Read the model definition and answer for the solid it produces. Units are mm, in the model's axes. A direction names the side the tool comes from. Coordinates: 2 decimals unless noted, no trailing zeros. Order: outer loops, then holes, each group sorted by start corner. A loop starts at its lowest first (then second) coordinate and runs counter-clockwise, first axis right, second up. Notation, with made-up numbers: (61.25, 48.5) - (83.25, 48.5) arc R28 ccw to (83.25, 80.5) - close; hole circle Ø10 at (20, -11.75). An arc over 180 degrees is marked (long way). Use one line per item in the form item = value. Start each with the question number.
from build123d import *

# Parameters (mm, degrees)
F1_W     = 57.62729
F1_H     = 2.417922
F2_DEPTH = 53.739645
F3_W     = 20.9051
F3_H     = 3.238531
F4_DEPTH = 25
F5_W     = 39.400994
F5_H     = 8.231058
F6_DEPTH = 25


with BuildPart() as f2:
    # F1 (on face) → F2 (new body)
    with BuildSketch(Plane.XZ):
        with Locations((0, 114.370458)):
            Rectangle(F1_W, F1_H)
    extrude(amount=F2_DEPTH)

    # F3 (on face) → F4 (cut)
    with BuildSketch(Plane.XY.offset(115.579419)):
        with Locations((0, -6.892247)):
            Rectangle(F3_W, F3_H)
    extrude(amount=-F4_DEPTH, mode=Mode.SUBTRACT)

    # F5 (on face) → F6 (cut)
    with BuildSketch(Plane.XZ):
        with Locations((0, -5.288288)):
            Rectangle(F5_W, F5_H)
    extrude(amount=F6_DEPTH, mode=Mode.SUBTRACT)


solid = f2.part
Q1. A cutting plane is placed at C-C (z = 113.65). Give the vertices of the cut face in (x, y), then the cut area to 3 significant figures.
Q2. Consider probe 1 along Y at (x, z) = (-8, 113.75); probe 2 along X at (y, z) = (-7, 115). Determine where each line is inside the solid, lowest interval first.
Q3. Which of the six approach directions +Z, -Z, +X, -X, +Y, -Y give full straight-line access (tool end or side, diameter ignored) to faces 4 (the flat face through (0, -26, 113.161)), 5 (the flat face through (0, -5.273, 114))?
Q4. For a pull along X with two mould halves and no side action, classify faces 1 (the flat face through (-28.814, -26, 114)), 2 (the flat face through (0, -53.74, 114)), 3 (the flat face through (10.453, -7, 114)) as +X half, -X half, draft (parallel to the pull), parting line (faces both ways), or undercut.
Q5. A cutting plane is placed at A-A (x = 0). Give the vertices of the cut face in (y, z).
Q6. A cutting plane is placed at B-B (y = -6). Give the vertices of the cut face in (x, z), then the cut area to 3 significant figures.
Result sheet:
q1.outline = (-28.81, -53.74) - (28.81, -53.74) - (28.81, 0) - (-28.81, 0) - close; hole (-10.45, -8.51) - (10.45, -8.51) - (10.45, -5.27) - (-10.45, -5.27) - close
q1.area = 3,030 mm^2
q2.probe_1 = -53.74 to -8.51, -5.27 to 0
q2.probe_2 = -28.81 to -10.45, 10.45 to 28.81
q3.face_4 = -Z, +X, -X, +Y, -Y
q3.face_5 = +Z, -Z
q4.face_1 = -X half
q4.face_2 = draft
q4.face_3 = undercut
q5.outline = (-53.74, 113.16) - (-8.51, 113.16) - (-8.51, 115.58) - (-53.74, 115.58) - close; (-5.27, 113.16) - (0, 113.16) - (0, 115.58) - (-5.27, 115.58) - close
q6.outline = (-28.81, 113.16) - (-10.45, 113.16) - (-10.45, 115.58) - (-28.81, 115.58) - close; (10.45, 113.16) - (28.81, 113.16) - (28.81, 115.58) - (10.45, 115.58) - close
q6.area = 88.8 mm^2
